The listing builds one solid part. Answer for the finished solid, in the listing's coordinates (mm). A direction names the side the tool comes from. Round coordinates to 2 decimals unless told otherwise and drop trailing zeros. Loops run counter-clockwise (first coordinate to the right, second up) from the corner with the lowest first, then second, coordinate; pieces in that order, holes last. Notation, with made-up numbers: (-8, 3) - (40, 3) arc R34 ccw to (40, 34) - close; hole circle Ø8 at (-2.75, 58). An arc over 180 degrees is marked (long way). Write item = value, one per line. Start each with the question number.
1) For a pull along Y with two mould halves and no side action, classify faces 4 (the flat face through (0, 30, 4)), 5 (the conical face through (19.879, 47.285, 3.972)), 6 (the cylindrical face through (24.2, 11.26, 4.16)), 7 (the flat face through (14, 0, 4)) as released by +Y, released by -Y, zero draft, split by the parting line, or undercut.
2) Straight lines are drawn through the part: line 1 along Y through (x, z) = (23, 4); line 2 along Z through (x, y) = (25.5, 12.5); line 3 along Y through (x, z) = (23, 5). For each, find the intervals that lie inside material, in ascending order.
3) Section A-A, the plane x = 25.75 is taken. Determine the outline of the cut face in (y, z), and give its area (3 significant figures).
4) A tool of negligible diameter and unlimited length cuts with its end or side. For faces 1 (the cylindrical face through (3.8, 46.26, 3.84)), 2 (the flat face through (14, 30, 0)), 3 (the cylindrical face through (24.2, 46.26, 4.16)), from which of +Z, -Z, +X, -X, +Y, -Y can it reach the whole face along a straight path? Write none if from no direction.
from build123d import *

# Parameters (mm, degrees)
SKETCH_1_W      = 28
SKETCH_1_H      = 60
EXTRUDE_1_DEPTH = 8
M3X0_5_1_D      = 2.5
M3X0_5_1_DEPTH  = 7.5
M3X0_5_1_TIP    = 0.751075774
M3X0_5_2_D      = 2.5
M3X0_5_2_DEPTH  = 7.5
M3X0_5_2_TIP    = 0.751075774


with BuildPart() as part:
    # ｽｹｯﾁ1 → ﾎﾞｽ - 押し出し1 (new body)
    with BuildSketch(Plane.XY):
        with Locations((14, 30)):
            Rectangle(SKETCH_1_W, SKETCH_1_H)
    extrude(amount=EXTRUDE_1_DEPTH)

    # M3x0.5 ねじ穴1
    with Locations(Plane(origin=(0, 47.5, 4), x_dir=(0, 0, -1), z_dir=(-1, 0, 0))):
        with Locations((0, 0), (0, 35)):
            Hole(M3X0_5_1_D / 2, depth=M3X0_5_1_DEPTH)
            with Locations((0, 0, -(M3X0_5_1_DEPTH + M3X0_5_1_TIP / 2))):  # 118° drill point
                Cone(0, M3X0_5_1_D / 2, M3X0_5_1_TIP, mode=Mode.SUBTRACT)

    # M3x0.5 ねじ穴2
    with Locations(Plane(origin=(28, 47.5, 4), x_dir=(0, 0, 1), z_dir=(1, 0, 0))):
        with Locations((0, 0), (0, 35)):
            Hole(M3X0_5_2_D / 2, depth=M3X0_5_2_DEPTH)
            with Locations((0, 0, -(M3X0_5_2_DEPTH + M3X0_5_2_TIP / 2))):  # 118° drill point
                Cone(0, M3X0_5_2_D / 2, M3X0_5_2_TIP, mode=Mode.SUBTRACT)


solid = part.part
Geometry check:
q1.face_4 = zero draft
q1.face_5 = undercut
q1.face_6 = undercut
q1.face_7 = released by -Y
q2.line_1 = 0 to 11.25, 13.75 to 46.25, 48.75 to 60
q2.line_2 = 0 to 2.75, 5.25 to 8
q2.line_3 = 0 to 11.75, 13.25 to 46.75, 48.25 to 60
q3.outline = (0, 0) - (60, 0) - (60, 8) - (0, 8) - close; hole circle Ø2.5 at (12.5, 4); hole circle Ø2.5 at (47.5, 4)
q3.area = 470 mm2
q4.face_1 = -X
q4.face_2 = -Z, +X, -X, +Y, -Y
q4.face_3 = +X
